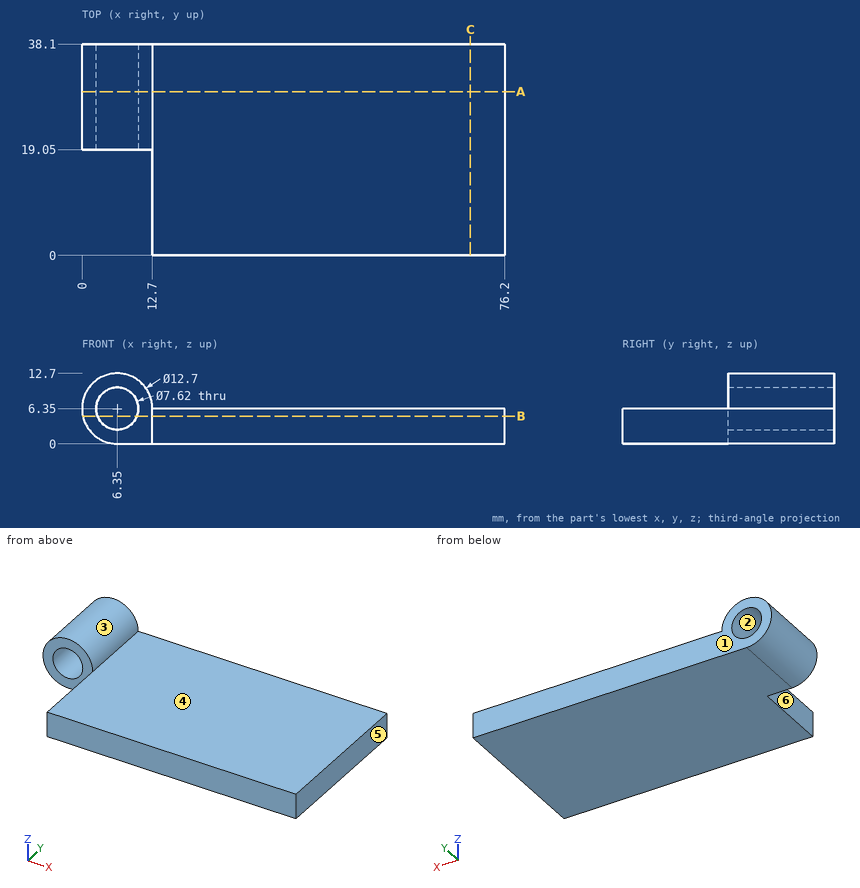
Could you check a few things on this drawing? It's one solid part, dimensions in mm from its lowest x, y, z. A direction names the side the tool comes from. Coordinates: 2 decimals unless noted, no trailing zeros. Write each loop counter-clockwise with the first axis right and the second up, starting at its lowest first coordinate (ties: lowest second). Pieces come first, ordered by that corner, then holes.
1) Which directions (+Z, -Z, +X, -X, +Y, -Y) give clear straight access to the entire face, cutting with the end or side of a thin tool? Please do the marked faces 4, 5 and 6.
Filled in:
face 4: +Z, +X, +Y, -Y
face 5: +Z, -Z, +X, +Y, -Y
face 6: +Z, -Z, -X, -Y
2) I'm going to push flat-ended pins straight in: pin 1 (5 mm diameter, centred on y = 7.5, z = 4, fed in from -X); pin 2 (2 mm diameter, centred on y = 24, z = 11.5, fed in from -X); pin 3 (1.5 mm diameter, centred on x = 44, y = 11, fed in from +Z). Where does each tip first touch, or does it pass through?
Filled in:
pin 1: stops at x = 12.7
pin 2: stops at x = 1.54
pin 3: stops at z = 6.35
3) Thinking about a two-plate mould opening in Z: for the marked faces 1, 2 and 3, which applies, +Z half, -Z half, draft (parallel to the pull), parting line (faces both ways), or undercut?
Filled in:
face 1: draft
face 2: undercut
face 3: parting line
4) If we section it at A-A (y = 29.5): List the corners of the cut face in (x, z) for me, plus the area to 3 significant figures.
Filled in:
outline: (6.35, 0) - (76.2, 0) - (76.2, 6.35) - (12.7, 6.35) arc R6.35 ccw (long way) to start; hole circle Ø7.62 at (6.35, 6.35)
area: 493 mm2
5) If we section it at C-C (x = 70): List the corners of the cut face in (y, z) for me.
Filled in:
outline: (0, 0) - (38.1, 0) - (38.1, 6.35) - (0, 6.35) - close
6) If I drill on line 1 (Z direction, x = 6.35, y = 23); line 2 (Z direction, x = 6, y = 24); line 3 (Z direction, x = 67.5, y = 26), over which ranges is the centre line in solid material (lowest first)?
Filled in:
line 1: z = 0 to 2.54, 10.16 to 12.7
line 2: z = 0.01 to 2.56, 10.14 to 12.69
line 3: z = 0 to 6.35
7) If we section it at B-B (z = 5): List the corners of the cut face in (x, y) for me.
Filled in:
outline: (0.15, 19.05) - (2.79, 19.05) - (2.79, 38.1) - (0.15, 38.1) - close; (9.91, 19.05) - (12.7, 19.05) - (12.7, 0) - (76.2, 0) - (76.2, 38.1) - (9.91, 38.1) - close
